```python
from build123d import *

# Parameters (mm, degrees)
F0_R     = 16.4465
F1_DEPTH = 25.4
F2_R     = 13.0175
F3_DEPTH = 48.26
F5_D     = 10.31875


with BuildPart() as f1:
    # F0 (on Top) → F1 (new body)
    with BuildSketch(Plane.XY):
        Circle(F0_R)
    extrude(amount=F1_DEPTH)

    # F2 (on face) → F3 (join)
    with BuildSketch(Plane.XY.offset(25.4)):
        Circle(F2_R)
    extrude(amount=F3_DEPTH)

    # F5 (through all)
    with Locations(Plane.XY.offset(73.66)):
        with Locations((0, 0)):
            Hole(F5_D / 2)


solid = f1.part
```
Could you check a few things on this model? Use its own coordinates, in mm. A direction names the side the tool comes from. Round coordinates to 2 decimals unless told otherwise and drop trailing zeros. Write each loop counter-clockwise with the first axis right and the second up, starting at its lowest first coordinate (ties: lowest second). Pieces come first, ordered by that corner, then holes. Notation, with made-up numbers: M -8,-32 L 25,-32 A3 ccw 25,-28 Z; hole C -27,8.5 d4. An arc over 180 degrees is marked long. Write each question's results on one line, items separated by ' | '. Start each with the question number.
1. Imagine slicing it at D-D on y = -12. List the corners of the cut face in (x, z) for me, and give its area (3 significant figures).
2. Imagine slicing it at C-C on z = 19. List the corners of the cut face in (x, y) for me, and give its area (3 significant figures).
3. Thinking about a two-plate mould opening in Y: for faces 1 (the face through (-1.695, 12.907, 49.192)), 2 (the face through (6, 0, 73.66)), 3 (the face through (1.118, -5.037, 36.314)), which applies, +Y half, -Y half, draft (parallel to the pull), parting line (faces both ways), or undercut?
4. On a 3-axis mill with a long thin cutter (end or side, diameter ignored), from which of +Z, -Z, +X, -X, +Y, -Y can I reach the whole of each face in a straight line? I mean faces 4 (the face through (-4, 4, 0)), 5 (the face through (-12.3, -4.8, 25.4)). Say none if no direction works.
5. I need wall thicknesses on L1, parallel to Y at x = 0, z = 55; L2, parallel to Z at x = -9.5, y = -9.5; L3, parallel to X at y = -2, z = 55. Which ranges of each line are inside material? Lowest first, please. Write a range as from..to.
6. I'm going to push flat-ended pins straight in: pin 1 Ø2 at (x, z) = (1.5, 16) entering from -Y; pin 2 Ø3 at (y, z) = (-11, 25.5) entering from +X; pin 3 Ø1 at (x, z) = (6.5, 40) entering from +Y. Where does each tip first touch, or does it pass through?
7. Imagine slicing it at A-A on y = 0. List the corners of the cut face in (x, z) for me, and give its area (3 significant figures).
Result sheet:
1) outline: M -11.25,0 L 11.25,0 L 11.25,25.4 L 5.05,25.4 L 5.05,73.66 L -5.05,73.66 L -5.05,25.4 L -11.25,25.4 Z | area: 1,060 mm^2
2) outline: C 0,0 d32.89; hole C 0,0 d10.32 | area: 766 mm^2
3) face 1: parting line | face 2: draft | face 3: undercut
4) face 4: -Z, +X, -X, +Y, -Y | face 5: +Z
5) L1: y = -13.02..-5.16, 5.16..13.02 | L2: z = 0..25.4 | L3: x = -12.86..-4.76, 4.76..12.86
6) pin 1: stops at y = -16.44 | pin 2: stops at x = 13.42 | pin 3: stops at y = 11.55
7) outline: M -16.45,0 L -5.16,0 L -5.16,73.66 L -13.02,73.66 L -13.02,25.4 L -16.45,25.4 Z; M 5.16,0 L 16.45,0 L 16.45,25.4 L 13.02,25.4 L 13.02,73.66 L 5.16,73.66 Z | area: 1,330 mm^2
